Study the drawing (mm; zero at the part's minimum x, y, z) and answer. A direction names the side the tool comes from. Coordinates: 2 decimals unless noted, no trailing zeros. Write each loop counter-clockwise with the first axis right and the second up, starting at its lowest first coordinate (ties: lowest second). Pieces come first, ordered by that corner, then holes. Notation, with made-up numbers: (-33, 86) -> (-19, 86) arc R33 ccw to (-19, 123) -> close; hole circle Ø11 at (-1, -37). An arc over 180 degrees is marked (long way). Write item = value, one per line. Start each with the question number.
1) Section D-D (x = 5) is taken. Determine the outline of the cut face in (y, z), plus the area to 3 significant figures.
2) For a pull along Y with two mould halves and no side action, classify the marked faces 1, 2 and 3 as released by +Y, released by -Y, zero draft, split by the parting line, or undercut.
3) Section A-A (x = 15) is taken. Determine the outline of the cut face in (y, z), plus the area to 4 significant figures.
4) Section B-B (y = 7.5) is taken. Determine the outline of the cut face in (x, z), plus the area to 4 significant figures.
5) Section C-C (z = 1.95) is taken. Determine the outline of the cut face in (x, y).
6) A tool of negligible diameter and unlimited length cuts with its end or side. For the marked faces 4 and 5, from which of +Z, -Z, +X, -X, +Y, -Y can it reach the whole face along a straight path? Write none if from no direction.
7) Find the intervals of material crossed by line 1 along Y through (x, z) = (15, 1.85); line 2 along Z through (x, y) = (15.75, 1.5); line 3 along Y through (x, z) = (5, 0.85), in increasing order. Write a range as from..to.
8) Flat-ended cylindrical pins translate along their axes: pin 1 Ø8.5 at (x, y) = (15, 7.5) entering from -Z; pin 2 Ø6.5 at (x, y) = (15.5, 9.5) entering from +Z. Find the tip coordinate at first contact, or state that the pin passes through.
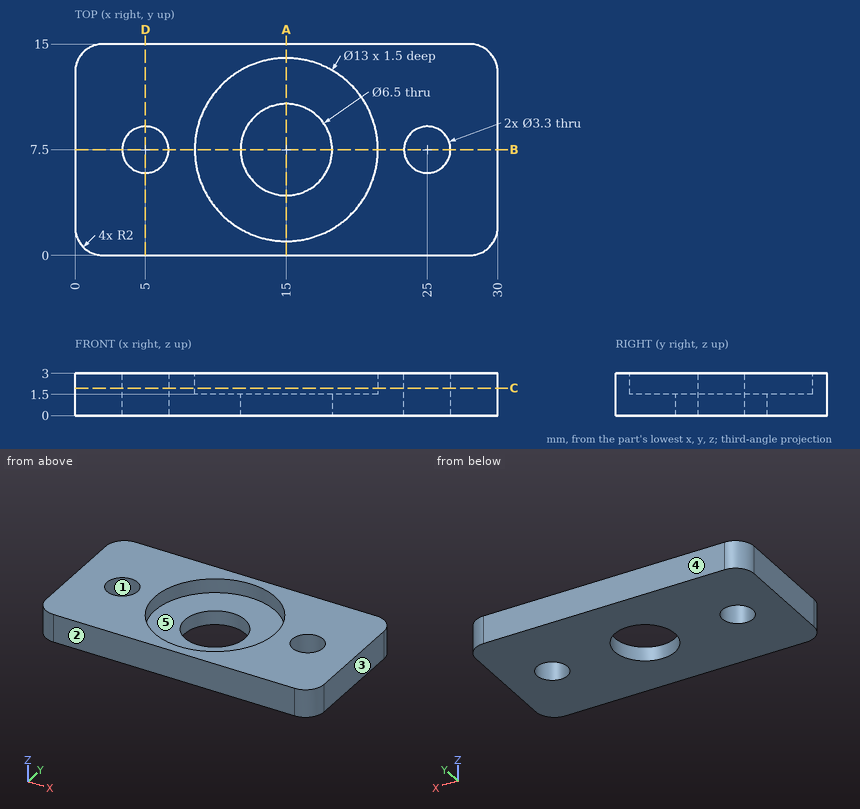
Answer key:
q1.outline = (0, 0) -> (5.85, 0) -> (5.85, 3) -> (0, 3) -> close; (9.15, 0) -> (15, 0) -> (15, 3) -> (9.15, 3) -> close
q1.area = 35.1 mm^2
q2.face_1 = undercut
q2.face_2 = released by -Y
q2.face_3 = zero draft
q3.outline = (0, 0) -> (4.25, 0) -> (4.25, 1.5) -> (1, 1.5) -> (1, 3) -> (0, 3) -> close; (10.75, 0) -> (15, 0) -> (15, 3) -> (14, 3) -> (14, 1.5) -> (10.75, 1.5) -> close
q3.area = 15.75 mm^2
q4.outline = (0, 0) -> (3.35, 0) -> (3.35, 3) -> (0, 3) -> close; (6.65, 0) -> (11.75, 0) -> (11.75, 1.5) -> (8.5, 1.5) -> (8.5, 3) -> (6.65, 3) -> close; (18.25, 0) -> (23.35, 0) -> (23.35, 3) -> (21.5, 3) -> (21.5, 1.5) -> (18.25, 1.5) -> close; (26.65, 0) -> (30, 0) -> (30, 3) -> (26.65, 3) -> close
q4.area = 40.95 mm^2
q5.outline = (0, 2) arc R2 ccw to (2, 0) -> (28, 0) arc R2 ccw to (30, 2) -> (30, 13) arc R2 ccw to (28, 15) -> (2, 15) arc R2 ccw to (0, 13) -> close; hole circle Ø3.3 at (5, 7.5); hole circle Ø13 at (15, 7.5); hole circle Ø3.3 at (25, 7.5)
q6.face_4 = +Z, -Z, +X, -X, +Y
q6.face_5 = +Z
q7.line_1 = 0..1, 14..15
q7.line_2 = 0..1.5
q7.line_3 = 0..5.85, 9.15..15
q8.pin_1 = 0
q8.pin_2 = 1.5
